Autodesk Inventor part; units mm, degrees
ref_plane "YZ Plane" through (0, 0, 0) normal (1, 0, 0) x (0, 1, 0)
ref_plane "XZ Plane" through (0, 0, 0) normal (0, 1, 0) x (-1, 0, 0)
ref_plane "XY Plane" through (0, 0, 0) normal (0, 0, 1) x (1, 0, 0)
ref_plane "Work Plane1" through (0, 0, 0) normal (0, 0, 1) x (1, 0, 0)
sketch "Sketch1" plane through (0, 0, 0) normal (0, 0, 1) x (1, 0, 0)
  circle A0 centre (0, 25) radius 1.95 construction
  circle A1 centre (-25, 0) radius 1.95 construction
  circle A2 centre (-25, -25) radius 1.95 construction
  circle A3 centre (25, 25) radius 1.95 construction
  circle A4 centre (25, -25) radius 1.95 construction
  circle A5 centre (-25, 25) radius 1.95 construction
  circle A6 centre (25, 0) radius 1.95 construction
  circle A7 centre (0, -25) radius 1.95 construction
  line L0 (-28, 30) -> (-30, 28) construction
  line L1 (-30, 28) -> (-30, -28) construction
  line L2 (-30, -28) -> (-28, -30) construction
  line L3 (-28, -30) -> (28, -30) construction
  line L4 (28, -30) -> (30, -28) construction
  line L5 (30, -28) -> (30, 28) construction
  line L6 (30, 28) -> (28, 30) construction
  line L7 (28, 30) -> (-28, 30) construction
  circle A8 centre (35, -56) radius 1 construction
  circle A9 centre (5, -48.5) radius 1 construction
  circle A10 centre (5, -64.5) radius 1.0474 construction
  circle A11 centre (-5, -64.5) radius 1 construction
  circle A12 centre (-5, -56) radius 1 construction
  circle A13 centre (-5, -48.5) radius 1 construction
  circle A14 centre (5, -56) radius 1 construction
  circle A15 centre (35, -48) radius 1 construction
  circle A16 centre (35, -64) radius 1 construction
  line L8 (38, -40) -> (38, -72) construction
  line L9 (38, -40) -> (-10, -40) construction
  line L10 (-10, -72) -> (-10, -40) construction
  line L11 (38, -72) -> (-10, -72) construction
  line L12 (38, -71) -> (38, -41) construction
  line L13 (38, -71) -> (48, -71) construction
  line L14 (48, -41) -> (48, -71) construction
  line L15 (38, -41) -> (48, -41) construction
  line L16 (56, -75) -> (-52.5, -75)
  line L17 (-52.5, -75) -> (-52.5, -30)
  line L18 (-52.5, -30) -> (56, -30)
  line L19 (56, -30) -> (56, -75)
  line L20 (-40, -41.1445) -> (-40, -68) construction
  line L21 (-41, -39.0927) -> (-41, -47.7587) construction
  line L22 (-41, -39.0927) -> (-46.5, -39.0927) construction
  line L23 (-46.5, -47.7587) -> (-46.5, -39.0927) construction
  line L24 (-41, -47.7587) -> (-46.5, -47.7587) construction
  line L25 (-41, -60.5) -> (-41, -64) construction
  line L26 (-41, -60.5) -> (-46.5, -60.5) construction
  line L27 (-46.5, -64) -> (-46.5, -60.5) construction
  line L28 (-41, -64) -> (-46.5, -64) construction
  line L29 (64, 30) -> (-96, 30)
  line L30 (-96, 30) -> (-96, -80)
  line L31 (-96, -80) -> (64, -80)
  line L32 (64, -80) -> (64, 30)
  line L33 (20, -20) -> (-20, -20)
  line L34 (-20, -20) -> (-20, 20)
  line L35 (-20, 20) -> (20, 20)
  line L36 (20, 20) -> (20, -20)
  line L37 (20, -20) -> (-20, 20) construction
  line L38 (-20, -20) -> (20, 20) construction
  line L39 (-52.5, -30) -> (-30, -30)
  line L40 (-30, -30) -> (-30, -25)
  line L41 (-30, -25) -> (-52.5, -25)
  line L42 (-52.5, -25) -> (-52.5, -30)
  point P0 (0, 0)
  dimension "d1" = 3
  dimension "d2" = 8
  dimension "d4" = 6
  dimension "d5" = 160
  dimension "d6" = 110
  dimension "d7" = 8
  dimension "d19" = 40
  dimension "d20" = 40
  dimension "d28" = 5
  dimension "d29" = 0
extrude "Extrusion1" add sketch "Sketch1" along normal blind 10
sketch "Sketch2" plane through (0, 0, 10) normal (0, 0, 1) x (1, 0, 0)
  line L0 (-30, -30) -> (56, -30)
  line L1 (56, -30) -> (56, -75)
  line L2 (56, -75) -> (-52.5, -75)
  line L3 (64, 30) -> (-96, 30)
  line L4 (-96, 30) -> (-96, -80)
  line L5 (-96, -80) -> (64, -80)
  line L6 (64, -80) -> (64, 30)
  line L7 (20, -20) -> (20, 20)
  line L8 (-20, -20) -> (20, -20)
  line L9 (20, -20) -> (20, 20)
  line L10 (20, 20) -> (-20, 20)
  line L11 (-20, 20) -> (-20, -20)
  line L12 (-20, -20) -> (20, 20) construction
  line L13 (20, -20) -> (-20, 20) construction
  line L14 (-52.5, -25) -> (-30, -25)
  line L15 (-30, -25) -> (-30, -30)
  line L16 (-52.5, -75) -> (-52.5, -25)
  point P0 (0, 0)
extrude "Extrusion2" add sketch "Sketch2" along normal blind 4 contours L0 L1 L2 L16 L14 L15 | L6 L5 L4 L3
sketch "Sketch3" plane through (0, 0, 14) normal (0, 0, 1) x (1, 0, 0)
  circle A0 centre (0, 25) radius 1.95 construction
  circle A1 centre (-25, 0) radius 1.95 construction
  circle A2 centre (-25, -25) radius 1.95 construction
  circle A3 centre (25, 25) radius 1.95 construction
  circle A4 centre (25, -25) radius 1.95 construction
  circle A5 centre (-25, 25) radius 1.95 construction
  circle A6 centre (25, 0) radius 1.95 construction
  circle A7 centre (0, -25) radius 1.95 construction
  line L0 (-28, 30) -> (-30, 28) construction
  line L1 (-30, 28) -> (-30, -28) construction
  line L2 (-30, -28) -> (-28, -30) construction
  line L3 (-28, -30) -> (28, -30) construction
  line L4 (28, -30) -> (30, -28) construction
  line L5 (30, -28) -> (30, 28) construction
  line L6 (30, 28) -> (28, 30) construction
  line L7 (28, 30) -> (-28, 30) construction
  point P0 (0, 0)
hole "Hole1" at (25, 25, 14) at (0, 25, 14) at (-25, 25, 14) at (-25, 0, 14) at (-25, -25, 14) at (0, -25, 14) at (25, -25, 14) at (25, 0, 14) direction (0, 0, -1) diameter 3.3 end through all counterbore diameter 8 counterbore depth 5
sketch "Sketch4" plane through (0, 0, 0) normal (0, 0, -1) x (-1, 0, 0)
  line L0 (52.5, -75) -> (-56, -75) construction
  line L1 (-56, -75) -> (-56, -30) construction
  line L2 (-56, -30) -> (30, -30) construction
  line L3 (20, 20) -> (20, -20) construction
  line L4 (20, -20) -> (-20, -20) construction
  line L5 (-20, -20) -> (-20, 20) construction
  line L6 (-20, 20) -> (20, 20) construction
  line L7 (-64, 30) -> (96, 30) construction
  line L8 (-64, -80) -> (-64, 30) construction
  line L9 (96, -80) -> (-64, -80) construction
  line L10 (96, 30) -> (96, -80) construction
  line L11 (60.9313, -70.255) -> (60.9313, -41.3875) construction
  line L12 (60.9313, -41.3875) -> (85.9313, -55.8212) construction
  line L13 (85.9313, -55.8212) -> (60.9313, -70.255) construction
  line L14 (96, 30) -> (96, -80) construction
  line L15 (30, -30) -> (30, -25)
  line L16 (30, -25) -> (52.5, -25)
  line L17 (52.5, -25) -> (52.5, -75)
  point P0 (0, 0)
  point P1 (69.2646, -55.8212)
  dimension "d30" = 25
hole "Hole2" at (-60.9313, -41.3875, 0) at (-85.9313, -55.8212, 0) at (-60.9313, -70.255, 0) direction (0, 0, 1) diameter 2.8 depth 12 tip angle 118 counterbore diameter 8 counterbore depth 4
properties part number "cellSTORM_Base_v0"
Here's how the part is built. I have some questions about the finished solid (model axes, mm). A direction names the side the tool comes from. Give positions to 0.01 mm unless a question says otherwise; leave off trailing zeros. Loops run counter-clockwise (first coordinate to the right, second up) from the corner with the lowest first, then second, coordinate; pieces in that order, holes last. Notation, with made-up numbers: M -20,71 L 26,71 A18 ccw 26,77 Z; hole C -32.75,28 d6. An arc over 180 degrees is marked long. Put each result on its own line as item: value. Start each with the question number.
(1) I want a section at B-B on y = 0. Please give me the cut outline in (x, z).
(2) I need wall thicknesses on line 1 along Y through (x, z) = (-25, 11.45); line 2 along X through (y, z) = (-25, 12.5); line 3 along Y through (x, z) = (-17.5, 5.5). Which ranges of each line are inside material? Lowest first, please. Write a range as [from, to].
(3) I want a section at A-A on x = 25. State how many separate pieces and enclosed holes the cut face has, then the cut area to 3 significant figures.
(4) Will these pins go through, and if not, where does the flat tip stop? pin 1 Ø2.5 at (x, y) = (-25.5, -1.5) entering from +Z; pin 2 Ø25 at (x, y) = (22.5, -54) entering from -Z; pin 3 Ø2 at (x, y) = (0, -25) entering from -Z.
(5) I want a section at C-C on y = 25. Please give me the cut outline in (x, z), then the cut area to 3 significant figures.
(6) For faces 1 (the flat face through (0, 20, 7)), 2 (the cylindrical face through (-28.966, -24.479, 11.465)), 3 (the flat face through (3, -75, 5)), which set-ups out of +Z, -Z, +X, -X, +Y, -Y let a thin tool reach every point of the face, with its end or its side?
Answer block:
1. outline: M -96,0 L -26.65,0 L -26.65,9 L -29,9 L -29,14 L -96,14 Z; M -23.35,0 L -20,0 L -20,14 L -21,14 L -21,9 L -23.35,9 Z; M 20,0 L 23.35,0 L 23.35,9 L 21,9 L 21,14 L 20,14 Z; M 26.65,0 L 64,0 L 64,14 L 29,14 L 29,9 L 26.65,9 Z
2. line 1: [-80, -29], [-21, -4], [4, 21], [29, 30]
2. line 2: [-96, -29], [-21, -4], [4, 21], [29, 64]
2. line 3: [-80, -75], [-30, -20], [20, 30]
3. separate pieces: 4
3. enclosed holes: 0
3. area: 881 mm^2
4. pin 1: z = 9
4. pin 2: z = 10
4. pin 3: through
5. outline: M -96,0 L -26.65,0 L -26.65,9 L -29,9 L -29,14 L -96,14 Z; M -23.35,0 L -1.65,0 L -1.65,9 L -4,9 L -4,14 L -21,14 L -21,9 L -23.35,9 Z; M 1.65,0 L 23.35,0 L 23.35,9 L 21,9 L 21,14 L 4,14 L 4,9 L 1.65,9 Z; M 26.65,0 L 64,0 L 64,14 L 29,14 L 29,9 L 26.65,9 Z
5. area: 2,030 mm^2
6. face 1: +Z, -Z
6. face 2: +Z
6. face 3: -Z
